Design review of the part built by this model. Coordinates are the model's own, in mm. A direction names the side the tool comes from. Coordinates: 2 decimals unless noted, no trailing zeros. Order: outer loops, then holes, each group sorted by start corner. A loop starts at its lowest first (then second) coordinate and runs counter-clockwise, first axis right, second up. Notation, with made-up numbers: (87.5, 26) -> (139.5, 26) arc R32 cw to (139.5, 64) -> close; hole circle Ø10 at (82.5, 65.5). An arc over 180 degrees is marked (long way). Write item = value, one per line.
```python
from build123d import *

# Parameters (mm, degrees)
CROQUIS1_W              = 750
CROQUIS1_H              = 1700
SALIENTE_EXTRUIR1_DEPTH = 700
REDONDEO1_R             = 10
CROQUIS2_R              = 40
SALIENTE_EXTRUIR2_DEPTH = 24
CROQUIS3_R              = 46
SALIENTE_EXTRUIR3_DEPTH = 10
REDONDEO2_R             = 5


with BuildPart() as part:
    # Croquis1 → Saliente-Extruir1 (new body)
    with BuildSketch(Plane.XY):
        with Locations((375, -850)):
            Rectangle(CROQUIS1_W, CROQUIS1_H)
    extrude(amount=SALIENTE_EXTRUIR1_DEPTH)

    # Redondeo1
    redondeo1_edges = [part.edges().sort_by_distance(p)[0] for p in [
        (750, -850, 700),
        (375, 0, 700),
        (0, -850, 700),
        (375, 0, 0),
        (750, -850, 0),
        (0, -850, 0),
        (0, 0, 350),
        (750, 0, 350),
    ]]
    fillet(redondeo1_edges, radius=REDONDEO1_R)

    # Croquis2 → Saliente-Extruir2 (add)
    with BuildSketch(Plane.XY.offset(700)):
        with Locations((130, -1610)):
            Circle(CROQUIS2_R)
    extrude(amount=SALIENTE_EXTRUIR2_DEPTH)

    # Croquis3 → Saliente-Extruir3 (add)
    with BuildSketch(Plane.XY.offset(724)):
        with Locations((130, -1610)):
            Circle(CROQUIS3_R)
    extrude(amount=-SALIENTE_EXTRUIR3_DEPTH)

    # Redondeo2
    redondeo2_edges = [part.edges().sort_by_distance(p)[0] for p in [
        (84, -1610, 724),
    ]]
    fillet(redondeo2_edges, radius=REDONDEO2_R)


solid = part.part
```
(1) We need section A-A (x = 130). Write out the cut boundary in (y, z).
Report:
outline = (-1700, 0) -> (-10, 0) arc R10 ccw to (0, 10) -> (0, 690) arc R10 ccw to (-10, 700) -> (-1570, 700) -> (-1570, 714) -> (-1564, 714) -> (-1564, 719) arc R5 ccw to (-1569, 724) -> (-1651, 724) arc R5 ccw to (-1656, 719) -> (-1656, 714) -> (-1650, 714) -> (-1650, 700) -> (-1700, 700) -> close
(2) The part is to be moulded in two halves that separate along Z. For faces 3 (the flat face through (116, -1572, 714)), 4 (the flat face through (0, -867, 345)), 5 (the flat face through (129, -1609, 724)), 6 (the cylindrical face through (124.79, -1570.34, 706.9)), say which applies: released by +Z, released by -Z, zero draft, split by the parting line, or undercut.
Report:
face_3 = undercut
face_4 = zero draft
face_5 = released by +Z
face_6 = undercut
(3) We need section D-D (x = 532.5). Write out the cut boundary in (y, z), and give its area (3 significant figures).
Report:
outline = (-1700, 0) -> (-10, 0) arc R10 ccw to (0, 10) -> (0, 690) arc R10 ccw to (-10, 700) -> (-1700, 700) -> close
area = 1,190,000 mm²
(4) For faces 1 (the flat face through (370, -1700, 345)), 2 (the cylindrical face through (120, -1654.9, 716.5)), list the 3-axis set-ups (+Z, -Z, +X, -X, +Y, -Y) from which the entire face can be reached by the end or side of a thin tool; tool diameter is ignored.
Report:
face_1 = +Z, -Z, +X, -X, -Y
face_2 = +Z
(5) We need section C-C (y = -931.5). Write out the cut boundary in (x, z).
Report:
outline = (0, 10) arc R10 ccw to (10, 0) -> (740, 0) arc R10 ccw to (750, 10) -> (750, 690) arc R10 ccw to (740, 700) -> (10, 700) arc R10 ccw to (0, 690) -> close
(6) We need section B-B (y = -1610). Write out the cut boundary in (x, z), and give its area (3 significant figures).
Report:
outline = (0, 10) arc R10 ccw to (10, 0) -> (740, 0) arc R10 ccw to (750, 10) -> (750, 690) arc R10 ccw to (740, 700) -> (170, 700) -> (170, 714) -> (176, 714) -> (176, 719) arc R5 ccw to (171, 724) -> (89, 724) arc R5 ccw to (84, 719) -> (84, 714) -> (90, 714) -> (90, 700) -> (10, 700) arc R10 ccw to (0, 690) -> close
area = 527,000 mm²
(7) For L1, parallel to Z at x = 354, y = -1290, list the stretches that pass through material, from the lowest coordinate up.
Report:
L1 = 0 to 700
(8) Insertion check: pin 1 (6 mm diameter, centred on x = 234.5, y = -1141.5, fed in from +Z). The pin has a flat end and moves straight along its axis. Give the tip position at first contact, or say it passes through.
Report:
pin_1 = 700
